Check sheet for the modelled part. Datum: model origin and axes. Units: mm. Face numbers are marked on the shaded views. A direction names the side the tool comes from. Give positions to 0.01 mm unless a question says otherwise; leave off trailing zeros. Order: outer loops, then holes, each group sorted by start corner. A loop starts at its lowest first (then second) coordinate and runs counter-clockwise, first axis right, second up. Notation, with made-up numbers: (15, 60.5) -> (40, 60.5) arc R16 ccw to (40, 64.5) -> close; hole circle Ø1 at (-22, 59). An arc over 180 degrees is marked (long way). Answer in a Markdown table with one row per item. Add a question column.
(1) Go/stop test with flat-tipped pins: pin 1 (1 mm diameter, centred on x = 19, z = 3, fed in from -Y); pin 2 (6 mm diameter, centred on x = 16.5, y = -1, fed in from -Z); pin 3 (1 mm diameter, centred on x = 12.5, z = 5.5, fed in from +Y). Record where each tip stops, or that it passes through.
(2) Set-up check for the marked faces 5, 6 and 7: record each of +Z, -Z, +X, -X, +Y, -Y from which the full face is reachable in a straight line by a thin tool's end or side.
(3) Cross-section at C-C (y = 6). Record the cut outline in (x, z), then the cut area to 3 significant figures.
(4) Thickness scan on L1, parallel to Z at x = 20, y = 6.25; L2, parallel to Y at x = 14.25, z = 6.5; L3, parallel to Y at x = 15.25, z = 3.5. Record the ranges inside material, lowest first. Write a range as [from, to].
(5) Cross-section at B-B (x = 8). Record the cut outline in (y, z), then the cut area to 3 significant figures.
(6) Release check for a two-part mould opening along Y. For the marked faces 1, 2, 3 and 4 record: released by +Y, released by -Y, zero draft, split by the parting line, or undercut.
(7) Cross-section at D-D (x = 20.75). Record the cut outline in (y, z).
(8) Cross-section at A-A (z = 0.75). Record the cut outline in (x, y), then the cut area to 3 significant figures.
```python
from build123d import *

# Parameters (mm, degrees)
F1_DEPTH      = 25
F2_R          = 2.5
F4_DEPTH      = 6.9152135624
F4_DEPTH_BACK = 6.9152135624


with BuildPart() as f1:
    # F0 (on Right) → F1 (new body)
    with BuildSketch(Plane.YZ):
        with BuildLine():
            Line((-6.5, 0), (-4.7958315233, 0))
            ThreePointArc((-4.7958315233, 0), (0, 1), (4.7958315233, 0))
            Line((4.7958315233, 0), (6.5, 0))
            ThreePointArc((6.5, 0), (6.9142135624, 1), (6.5, 2))
            Line((6.5, 2), (2, 2))
            Line((2, 2), (1.2065285868, 6.5))
            ThreePointArc((1.2065285868, 6.5), (0, 7.5123976922), (-1.2065285868, 6.5))
            Line((-1.2065285868, 6.5), (-2, 2))
            Line((-2, 2), (-6.5, 2))
            ThreePointArc((-6.5, 2), (-6.9142135624, 1), (-6.5, 0))
        make_face()
    extrude(amount=F1_DEPTH)

    # F2
    f2_edges = [f1.edges().sort_by_distance(p)[0] for p in [
        (12.5, 2, 2),
        (12.5, -2, 2),
    ]]
    fillet(f2_edges, radius=F2_R)

    # F3 (on Front) → F4 (cut, two sides)
    with BuildSketch(Plane.XZ) as f4_sk:
        Polygon((8, 11.9143333792), (30, -0.787372543), (30, 11.9143333792), align=None)
    extrude(amount=-F4_DEPTH, mode=Mode.SUBTRACT)
    extrude(f4_sk.sketch, amount=F4_DEPTH_BACK, mode=Mode.SUBTRACT)


solid = f1.part
```
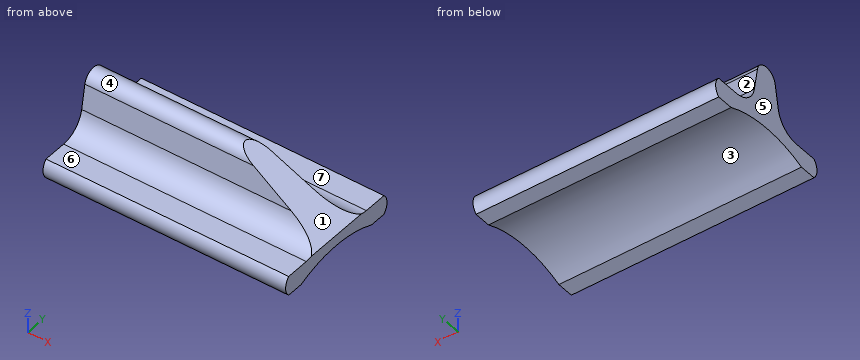
Answer below:
| question | item | result |
|---|---|---|
| 1 | pin 1 | stops at y = -2.6 |
| 1 | pin 2 | stops at z = 0.31 |
| 1 | pin 3 | stops at y = 1.47 |
| 2 | face 5 | +Z, -Z, -X, +Y, -Y |
| 2 | face 6 | +Z, +X, -X, -Y |
| 2 | face 7 | +Z, +X, -X, +Y |
| 3 | outline | (0, 0) -> (25, 0) -> (25, 2) -> (0, 2) -> close |
| 3 | area | 50.0 mm² |
| 4 | L1 | z = [0, 2] |
| 4 | L2 | y = [-1.21, 1.21] |
| 4 | L3 | y = [-1.81, 1.81] |
| 5 | outline | (-6.5, 0) -> (-4.8, 0) arc R12 cw to (4.8, 0) -> (6.5, 0) arc R1.41 ccw to (6.5, 2) -> (4.1, 2) arc R2.5 cw to (1.64, 4.07) -> (1.21, 6.5) arc R1.23 ccw to (-1.21, 6.5) -> (-1.64, 4.07) arc R2.5 cw to (-4.1, 2) -> (-6.5, 2) arc R1.41 ccw to start |
| 5 | area | 38.7 mm² |
| 6 | face 1 | zero draft |
| 6 | face 2 | released by +Y |
| 6 | face 3 | undercut |
| 6 | face 4 | split by the parting line |
| 7 | outline | (-6.5, 0) -> (-4.8, 0) arc R12 cw to (4.8, 0) -> (6.5, 0) arc R1.41 ccw to (6.5, 2) -> (4.1, 2) arc R2.5 cw to (1.64, 4.07) -> (1.55, 4.55) -> (-1.55, 4.55) -> (-1.64, 4.07) arc R2.5 cw to (-4.1, 2) -> (-6.5, 2) arc R1.41 ccw to start |
| 8 | outline | (0, -6.89) -> (25, -6.89) -> (25, -2.44) -> (0, -2.44) -> close; (0, 2.44) -> (25, 2.44) -> (25, 6.89) -> (0, 6.89) -> close |
| 8 | area | 223 mm² |
